from build123d import *

# Parameters (mm, degrees)
F1_DEPTH = 3.048


with BuildPart() as f1:
    # F0 (on Front) → F1 (new body)
    with BuildSketch(Plane.XZ):
        with BuildLine():
            Line((-19.05, 50.8), (-50.8, 50.8))
            ThreePointArc((-50.8, 50.8), (-36.455858, 15.421894), (-1.524, 0.022865))
            Line((-1.524, 0.022865), (-1.524, 25.4))
            Line((-1.524, 25.4), (1.524, 25.4))
            Line((1.524, 25.4), (1.524, 0.022865))
            ThreePointArc((1.524, 0.022865), (36.455858, 15.421894), (50.8, 50.8))
            Line((50.8, 50.8), (19.05, 50.8))
            Line((19.05, 50.8), (19.05, 53.848))
            Line((19.05, 53.848), (6.35, 53.848))
            Line((6.35, 53.848), (6.35, 50.8))
            Line((6.35, 50.8), (-6.35, 50.8))
            Line((-6.35, 50.8), (-6.35, 53.848))
            Line((-6.35, 53.848), (-19.05, 53.848))
            Line((-19.05, 53.848), (-19.05, 50.8))
        make_face()
    extrude(amount=F1_DEPTH)


solid = f1.part
The listing builds one solid part. Answer for the finished solid, in the listing's coordinates (mm). A direction names the side the tool comes from. Give positions to 0.01 mm unless a question says otherwise; leave off trailing zeros. Write each loop counter-clockwise with the first axis right and the second up, starting at its lowest first coordinate (ties: lowest second). Pieces come first, ordered by that corner, then holes. Notation, with made-up numbers: (44.25, 13) -> (62.25, 13) arc R17 cw to (62.25, 29) -> close; hole circle Ø10 at (-13, 79.5). An arc over 180 degrees is marked (long way). Use a Markdown table: item, result.
(1) Find the intervals of material crossed by probe 1 along X at (y, z) = (-0.9, 23); probe 2 along X at (y, z) = (-0.75, 13); probe 3 along Z at (x, y) = (-7, -2.6), in increasing order. Write a range as from..to.
Return value:
| item | result |
|---|---|
| probe 1 | -42.52..-1.52, 1.52..42.52 |
| probe 2 | -33.94..-1.52, 1.52..33.94 |
| probe 3 | 0.48..53.85 |
(2) Determine the mould class of faces 1 (the flat face through (35, -2, 50.8)), 2 (the cylindrical face through (36.07, -1.5, 15.03)), 3 (the flat face through (6.35, -2, 52)) for opening direction X: released by +X, released by -X, zero draft, split by the parting line, or undercut.
Return value:
| item | result |
|---|---|
| face 1 | zero draft |
| face 2 | released by +X |
| face 3 | undercut |
(3) Section A-A, the plane y = -2.5 is taken. Determine the outline of the cut face in (x, z).
Return value:
| item | result |
|---|---|
| outline | (-50.8, 50.8) arc R50.8 ccw to (-1.52, 0.02) -> (-1.52, 25.4) -> (1.52, 25.4) -> (1.52, 0.02) arc R50.8 ccw to (50.8, 50.8) -> (19.05, 50.8) -> (19.05, 53.85) -> (6.35, 53.85) -> (6.35, 50.8) -> (-6.35, 50.8) -> (-6.35, 53.85) -> (-19.05, 53.85) -> (-19.05, 50.8) -> close |
(4) Flat-ended cylindrical pins translate along their axes: P1, Ø1.5, axis at y = -2, z = 22.5, coming from the +X side; P2, Ø0.9, axis at x = -40, y = -1, coming from the +Z side; P3, Ø1.5, axis at y = -1, z = 7.5, coming from the -X side. Find the tip coordinate at first contact, or state that the pin passes through.
Return value:
| item | result |
|---|---|
| P1 | x = 42.68 |
| P2 | z = 50.8 |
| P3 | x = -27.75 |
(5) For faces 4 (the flat face through (0, -2, 25.4)), 5 (the flat face through (19.05, -2, 52)), 6 (the flat face through (0, -2, 50.8)), determine the directions among +Z, -Z, +X, -X, +Y, -Y from which every point of the face is accessible in a straight line to the end or side of a thin tool.
Return value:
| item | result |
|---|---|
| face 4 | -Z, +Y, -Y |
| face 5 | +Z, +X, +Y, -Y |
| face 6 | +Z, +Y, -Y |
(6) Section D-D, the plane z = 29 is taken. Determine the outline of the cut face in (x, y), then the cut area to 3 significant figures.
Return value:
| item | result |
|---|---|
| outline | (-45.88, -3.05) -> (45.88, -3.05) -> (45.88, 0) -> (-45.88, 0) -> close |
| area | 280 mm2 |
(7) Section C-C, the plane x = 10 is taken. Determine the outline of the cut face in (y, z), then the cut area to 3 significant figures.
Return value:
| item | result |
|---|---|
| outline | (-3.05, 0.99) -> (0, 0.99) -> (0, 53.85) -> (-3.05, 53.85) -> close |
| area | 161 mm2 |
(8) Section B-B, the plane z = 21 is taken. Determine the outline of the cut face in (x, y).
Return value:
| item | result |
|---|---|
| outline | (-41.14, -3.05) -> (-1.52, -3.05) -> (-1.52, 0) -> (-41.14, 0) -> close; (1.52, -3.05) -> (41.14, -3.05) -> (41.14, 0) -> (1.52, 0) -> close |
